Work out the finished part from the listing and answer in its coordinate system (mm). Give positions to 0.01 mm unless a question says otherwise; leave off trailing zeros.
1) Given pin 1 Ø0.8 at (x, y) = (9.5, 13) entering from +Z, flat-ended and moving along its own axis, determine where the tip first touches the part or whether it passes through.
2) A straight line is drawn through the part: probe 1 along Z at (x, y) = (21, -2). Find the intervals that lie inside material, in ascending order.
3) Find section A-A (z = 0.3). Count the separate pieces of the cut face and the enclosed holes in it, plus the area to 3 significant figures.
```python
from build123d import *

# Parameters (mm, degrees)
F1_DEPTH = 0.2
F3_DEPTH = 0.4
F2_W     = 85
F2_H     = 1.5
F4_DEPTH = 0.2


with BuildPart() as f1:
    # F0 (on Top) → F1 (new body)
    with BuildSketch(Plane.XY):
        with BuildLine():
            ThreePointArc((42.5, 64), (41.474874, 66.474874), (39, 67.5))
            Line((39, 67.5), (-39, 67.5))
            ThreePointArc((-39, 67.5), (-41.474874, 66.474874), (-42.5, 64))
            Line((-42.5, 64), (-42.5, -64))
            ThreePointArc((-42.5, -64), (-41.474874, -66.474874), (-39, -67.5))
            Line((-39, -67.5), (39, -67.5))
            ThreePointArc((39, -67.5), (41.474874, -66.474874), (42.5, -64))
            Line((42.5, -64), (42.5, 64))
        make_face()
    extrude(amount=F1_DEPTH)

    # F0 (on Top) → F3 (join)
    with BuildSketch(Plane.XY):
        with BuildLine():
            ThreePointArc((42.5, 64), (41.474874, 66.474874), (39, 67.5))
            Line((39, 67.5), (-39, 67.5))
            ThreePointArc((-39, 67.5), (-41.474874, 66.474874), (-42.5, 64))
            Line((-42.5, 64), (-42.5, -64))
            ThreePointArc((-42.5, -64), (-41.474874, -66.474874), (-39, -67.5))
            Line((-39, -67.5), (39, -67.5))
            ThreePointArc((39, -67.5), (41.474874, -66.474874), (42.5, -64))
            Line((42.5, -64), (42.5, 64))
        make_face()
    extrude(amount=F3_DEPTH)

    # F2 (on face) → F4 (cut, through all)
    with BuildSketch(Plane.XY.offset(0.2)):
        with Locations((0, 12.75)):
            Rectangle(F2_W, F2_H)
        with Locations((0, 9.25)):
            Rectangle(F2_W, F2_H)
        with Locations((0, 5.75)):
            Rectangle(F2_W, F2_H)
        with Locations((0, -12.75)):
            Rectangle(F2_W, F2_H)
        with Locations((0, -9.25)):
            Rectangle(F2_W, F2_H)
        with Locations((0, -5.75)):
            Rectangle(F2_W, F2_H)
        with Locations((0, 2.25)):
            Rectangle(F2_W, F2_H)
        with Locations((0, -2.25)):
            Rectangle(F2_W, F2_H)
    extrude(amount=F4_DEPTH, mode=Mode.SUBTRACT)


solid = f1.part
```
Results:
1. pin 1: stops at z = 0.2
2. probe 1: z = 0 to 0.2
3. separate pieces: 9
3. enclosed holes: 0
3. area: 10,400 mm2
